Read the model definition and answer for the solid it produces. Units are mm, in the model's axes. Face numbers are marked on the shaded views. A direction names the side the tool comes from. Coordinates: 2 decimals unless noted, no trailing zeros. Loops run counter-clockwise (first coordinate to the right, second up) from the corner with the lowest first, then second, coordinate; pieces in that order, holes last. Notation, with made-up numbers: M 41,-9.75 L 88,-9.75 A30 cw 88,18.25 Z; hole C 40.25,0.5 d11. An arc over 180 degrees is marked long. Use one line per item in the form item = value. Start each with the question number.
1. The part is cut by section D-D (x = 0). Give the vertices of the cut face in (y, z), plus the area to 3 significant figures.
2. The part is cut by section A-A (z = 49). Give the vertices of the cut face in (x, y).
3. Find the intervals of material crossed by probe 1 along Y at (x, z) = (27.4, 53.4); probe 2 along Y at (x, z) = (-15.5, 53.85); probe 3 along Y at (x, z) = (29, 51.5), in increasing order. Write a range as [from, to].
4. A tool of negligible diameter and unlimited length cuts with its end or side. For the marked faces 1 and 2, from which of +Z, -Z, +X, -X, +Y, -Y can it reach the whole face along a straight path? Write none if from no direction.
5. The part is cut by section C-C (y = -19.5). Give the vertices of the cut face in (x, z), plus the area to 3 significant figures.
6. The part is cut by section B-B (x = -27.4). Give the vertices of the cut face in (y, z), plus the area to 3 significant figures.
7. Flat-ended cylindrical pins translate along their axes: pin 1 (3 mm diameter, centred on x = 20, z = 40, fed in from +Y); pin 2 (4 mm diameter, centred on x = 15.5, y = -50.5, fed in from -Z); pin 3 (2 mm diameter, centred on x = -5, y = -12, fed in from -Z). Find the tip coordinate at first contact, or state that the pin passes through.
8. For a pull along Y with two mould halves and no side action, classify the marked faces 3, 4, 5 and 6 as released by +Y, released by -Y, zero draft, split by the parting line, or undercut.
from build123d import *

# Parameters (mm, degrees)
SKETCH003_W     = 66.8
SKETCH003_H     = 42
SKETCH003_R     = 1.5
SKETCH003_R_2   = 13
PAD003_DEPTH    = 4
PAD003_FACE3_W  = 66.8
PAD003_FACE3_H  = 4
PAD004_DEPTH    = 0.6
PAD004_FACE19_W = 66.8
PAD004_FACE19_H = 4
PAD005_DEPTH    = 4
PAD005_FACE21_W = 4
PAD005_FACE21_H = 66.8
PAD006_DEPTH    = 20
PAD006_FACE1_W  = 66.8
PAD006_FACE1_H  = 4
PAD007_DEPTH    = 0.6
PAD007_FACE11_W = 66.8
PAD007_FACE11_H = 4
PAD008_DEPTH    = 4
PAD008_FACE28_W = 4
PAD008_FACE28_H = 66.8
PAD009_DEPTH    = 10
FILLET003_R     = 2


with BuildPart() as part:
    # Sketch003 → Pad003 (new body)
    with BuildSketch(Plane.XY):
        with Locations((0, -35)):
            Rectangle(SKETCH003_W, SKETCH003_H)
        with Locations((-27.4, -26)):
            Circle(SKETCH003_R, mode=Mode.SUBTRACT)
        with Locations((0, -35)):
            Circle(SKETCH003_R_2, mode=Mode.SUBTRACT)
        with Locations((27.4, -26)):
            Circle(SKETCH003_R, mode=Mode.SUBTRACT)
        with Locations((27.4, -44)):
            Circle(SKETCH003_R, mode=Mode.SUBTRACT)
        with Locations((-27.4, -44)):
            Circle(SKETCH003_R, mode=Mode.SUBTRACT)
        with Locations((-15.5, -50.5)):
            Circle(SKETCH003_R, mode=Mode.SUBTRACT)
        with Locations((15.5, -50.5)):
            Circle(SKETCH003_R, mode=Mode.SUBTRACT)
        with Locations((-15.5, -19.5)):
            Circle(SKETCH003_R, mode=Mode.SUBTRACT)
        with Locations((15.5, -19.5)):
            Circle(SKETCH003_R, mode=Mode.SUBTRACT)
    extrude(amount=PAD003_DEPTH)

    # Pad003 Face3 → Pad004 (add)
    with BuildSketch(Plane(origin=(0, -56, 2), x_dir=(-1, 0, 0), z_dir=(0, -1, 0))):
        Rectangle(PAD003_FACE3_W, PAD003_FACE3_H)
    extrude(amount=PAD004_DEPTH)

    # Pad004 Face19 → Pad005 (add)
    with BuildSketch(Plane(origin=(0, -56.6, 2), x_dir=(-1, 0, 0), z_dir=(0, -1, 0))):
        Rectangle(PAD004_FACE19_W, PAD004_FACE19_H)
    extrude(amount=PAD005_DEPTH)

    # Pad005 Face21 → Pad006 (add)
    with BuildSketch(Plane(origin=(0, -58.6, 0), x_dir=(0, -1, 0), z_dir=(0, 0, -1))):
        Rectangle(PAD005_FACE21_W, PAD005_FACE21_H)
    extrude(amount=PAD006_DEPTH)

    # Pad006 Face1 → Pad007 (add)
    with BuildSketch(Plane(origin=(0, -14, 2), x_dir=(1, 0, 0), z_dir=(0, 1, 0))):
        Rectangle(PAD006_FACE1_W, PAD006_FACE1_H)
    extrude(amount=PAD007_DEPTH)

    # Pad007 Face11 → Pad008 (add)
    with BuildSketch(Plane(origin=(0, -13.4, 2), x_dir=(1, 0, 0), z_dir=(0, 1, 0))):
        Rectangle(PAD007_FACE11_W, PAD007_FACE11_H)
    extrude(amount=PAD008_DEPTH)

    # Pad008 Face28 → Pad009 (add)
    with BuildSketch(Plane(origin=(0, -11.4, 0), x_dir=(0, -1, 0), z_dir=(0, 0, -1))):
        Rectangle(PAD008_FACE28_W, PAD008_FACE28_H)
    extrude(amount=PAD009_DEPTH)

    # Fillet003
    fillet003_edges = [part.edges().sort_by_distance(p)[0] for p in [
        (0, -60.6, -20),
        (0, -60.6, 4),
        (0, -9.4, 4),
        (0, -9.4, -10),
    ]]
    fillet(fillet003_edges, radius=FILLET003_R)


with BuildPart() as part_1:
    # Body001 placement: moved
    add(part.part.moved(Location((0, 0, 52))))


solid = part_1.part
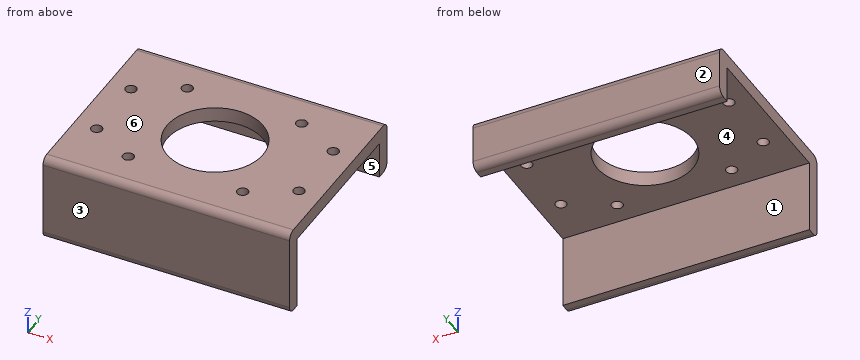
Computed values:
q1.outline = M -60.6,34 A2 ccw -58.6,32 L -56.6,32 L -56.6,52 L -48,52 L -48,56 L -58.6,56 A2 ccw -60.6,54 Z; M -22,52 L -13.4,52 L -13.4,42 L -11.4,42 A2 ccw -9.4,44 L -9.4,54 A2 ccw -11.4,56 L -22,56 Z
q1.area = 217 mm²
q2.outline = M -33.4,-60.6 L 33.4,-60.6 L 33.4,-56.6 L -33.4,-56.6 Z; M -33.4,-13.4 L 33.4,-13.4 L 33.4,-9.4 L -33.4,-9.4 Z
q3.probe_1 = [-60.6, -45.5], [-42.5, -27.5], [-24.5, -9.4]
q3.probe_2 = [-60.6, -52], [-49, -21], [-18, -9.4]
q3.probe_3 = [-60.6, -56.6], [-13.4, -9.4]
q4.face_1 = -Z, +X, -X
q4.face_2 = +Z, -Z, +X, -X, +Y
q5.outline = M -33.4,52 L -17,52 L -17,56 L -33.4,56 Z; M -14,52 L 14,52 L 14,56 L -14,56 Z; M 17,52 L 33.4,52 L 33.4,56 L 17,56 Z
q5.area = 243 mm²
q6.outline = M -60.6,34 A2 ccw -58.6,32 L -56.6,32 L -56.6,52 L -45.5,52 L -45.5,56 L -58.6,56 A2 ccw -60.6,54 Z; M -42.5,52 L -27.5,52 L -27.5,56 L -42.5,56 Z; M -24.5,52 L -13.4,52 L -13.4,42 L -11.4,42 A2 ccw -9.4,44 L -9.4,54 A2 ccw -11.4,56 L -24.5,56 Z
q6.area = 297 mm²
q7.pin_1 = -56.6
q7.pin_2 = 52
q7.pin_3 = 42
q8.face_3 = released by -Y
q8.face_4 = undercut
q8.face_5 = undercut
q8.face_6 = zero draft
